Design review of the part built by this model. Coordinates are the model's own, in mm. Face numbers are marked on the shaded views. A direction names the side the tool comes from. Give positions to 0.01 mm unless a question says otherwise; leave off trailing zeros. Write each loop counter-clockwise with the first axis right and the second up, starting at its lowest first coordinate (ties: lowest second). Pieces come first, ordered by that corner, then holes. Notation, with made-up numbers: (-13, 8) - (41, 8) arc R14 ccw to (41, 29) - close; hole circle Ø2 at (84, 80.5). An arc over 180 degrees is marked (long way). Use a Markdown table: item, result. Add a question column.
```python
from build123d import *

# Parameters (mm, degrees)
SKETCH1_R                                           = 35
BOSS_EXTRUDE1_DEPTH                                 = 12
BOSS_EXTRUDE2_START                                 = -4
SKETCH2_R                                           = 35
SKETCH2_R_2                                         = 17.5
BOSS_EXTRUDE2_DEPTH                                 = 4
SKETCH3_W                                           = 20
SKETCH3_H                                           = 20
BOSS_EXTRUDE3_DEPTH                                 = 5.5
CIRPATTERN1_COUNT                                   = 4
CUT_EXTRUDE1_REACH                                  = 123.475
SKETCH4_R                                           = 2.5
FILLET2_R                                           = 10
SKETCH5_R                                           = 35
SKETCH5_R_2                                         = 17.5
BOSS_EXTRUDE4_DEPTH                                 = 6
CSK_FOR_M3_COUNTERSUNK_FLAT_HEAD_SCREW1_D           = 3.4
CSK_FOR_M3_COUNTERSUNK_FLAT_HEAD_SCREW1_CSINK_D     = 6.3
CSK_FOR_M3_COUNTERSUNK_FLAT_HEAD_SCREW1_CSINK_ANGLE = 90
CHAMFER1_SIZE                                       = 1
CHAMFER2_SIZE                                       = 1


with BuildPart() as part:
    # Sketch1 → Boss-Extrude1 (new body)
    with BuildSketch(Plane.XY):
        with BuildLine():
            Line((43.874821937, -10), (85, -10))
            Line((85, -10), (85, 10))
            Line((85, 10), (43.874821937, 10))
            ThreePointArc((43.874821937, 10), (31.819805153, 31.819805153), (10, 43.874821937))
            Line((10, 43.874821937), (10, 85))
            Line((10, 85), (-10, 85))
            Line((-10, 85), (-10, 43.874821937))
            ThreePointArc((-10, 43.874821937), (-31.819805153, 31.819805153), (-43.874821937, 10))
            Line((-43.874821937, 10), (-85, 10))
            Line((-85, 10), (-85, -10))
            Line((-85, -10), (-43.874821937, -10))
            ThreePointArc((-43.874821937, -10), (-31.819805153, -31.819805153), (-10, -43.874821937))
            Line((-10, -43.874821937), (-10, -85))
            Line((-10, -85), (10, -85))
            Line((10, -85), (10, -43.874821937))
            ThreePointArc((10, -43.874821937), (31.819805153, -31.819805153), (43.874821937, -10))
        make_face()
        Circle(SKETCH1_R, mode=Mode.SUBTRACT)
    extrude(amount=BOSS_EXTRUDE1_DEPTH)

    # Sketch2 → Boss-Extrude2 (add)
    with BuildSketch(Plane.XY.offset(12).offset(BOSS_EXTRUDE2_START)):
        Circle(SKETCH2_R)
        Circle(SKETCH2_R_2, mode=Mode.SUBTRACT)
    extrude(amount=BOSS_EXTRUDE2_DEPTH)

    # Sketch3 → Boss-Extrude3 (add)
    with BuildSketch(Plane.XY):
        with Locations((0, 75)):
            Rectangle(SKETCH3_W, SKETCH3_H)
    boss_extrude3 = extrude(amount=-BOSS_EXTRUDE3_DEPTH)

    # CirPattern1: Boss-Extrude3 ×4 about axis
    cirpattern1_axis = Axis((0, 0, 0), (0, 0, 1))
    for i in range(1, CIRPATTERN1_COUNT):
        add(boss_extrude3.rotate(cirpattern1_axis, i * 360 / CIRPATTERN1_COUNT))

    # Sketch4 → Cut-Extrude1 (cut, up to next)
    with BuildSketch(Plane(origin=(0, 0, -5.5), x_dir=(-1, 0, 0), z_dir=(0, 0, -1)), mode=Mode.PRIVATE) as cut_extrude1_sk1:
        with Locations((0, 75)):
            Circle(SKETCH4_R)
    cut_extrude1_tool1 = extrude(cut_extrude1_sk1.sketch, amount=-CUT_EXTRUDE1_REACH, mode=Mode.PRIVATE) & part.part
    # Sketch4 → Cut-Extrude1 (cut, up to next)
    with BuildSketch(Plane(origin=(0, 0, -5.5), x_dir=(-1, 0, 0), z_dir=(0, 0, -1)), mode=Mode.PRIVATE) as cut_extrude1_sk2:
        with Locations((-75, 0)):
            Circle(SKETCH4_R)
    cut_extrude1_tool2 = extrude(cut_extrude1_sk2.sketch, amount=-CUT_EXTRUDE1_REACH, mode=Mode.PRIVATE) & part.part
    # Sketch4 → Cut-Extrude1 (cut, up to next)
    with BuildSketch(Plane(origin=(0, 0, -5.5), x_dir=(-1, 0, 0), z_dir=(0, 0, -1)), mode=Mode.PRIVATE) as cut_extrude1_sk3:
        with Locations((0, -75)):
            Circle(SKETCH4_R)
    cut_extrude1_tool3 = extrude(cut_extrude1_sk3.sketch, amount=-CUT_EXTRUDE1_REACH, mode=Mode.PRIVATE) & part.part
    # Sketch4 → Cut-Extrude1 (cut, up to next)
    with BuildSketch(Plane(origin=(0, 0, -5.5), x_dir=(-1, 0, 0), z_dir=(0, 0, -1)), mode=Mode.PRIVATE) as cut_extrude1_sk4:
        with Locations((75, 0)):
            Circle(SKETCH4_R)
    cut_extrude1_tool4 = extrude(cut_extrude1_sk4.sketch, amount=-CUT_EXTRUDE1_REACH, mode=Mode.PRIVATE) & part.part
    add(cut_extrude1_tool1.solids().sort_by_distance((0, 75, -5.5))[0], mode=Mode.SUBTRACT)
    add(cut_extrude1_tool2.solids().sort_by_distance((75, 0, -5.5))[0], mode=Mode.SUBTRACT)
    add(cut_extrude1_tool3.solids().sort_by_distance((0, -75, -5.5))[0], mode=Mode.SUBTRACT)
    add(cut_extrude1_tool4.solids().sort_by_distance((-75, 0, -5.5))[0], mode=Mode.SUBTRACT)

    # Fillet2
    fillet2_edges = [part.edges().sort_by_distance(p)[0] for p in [
        (10, -43.874821937, 6),
        (-10, -43.874821937, 6),
        (-43.874821937, -10, 6),
        (-43.874821937, 10, 6),
        (-10, 43.874821937, 6),
        (10, 43.874821937, 6),
        (43.874821937, 10, 6),
        (43.874821937, -10, 6),
    ]]
    fillet(fillet2_edges, radius=FILLET2_R)

    # Sketch5 → Boss-Extrude4 (add)
    with BuildSketch(Plane.XY.offset(12)):
        Circle(SKETCH5_R)
        Circle(SKETCH5_R_2, mode=Mode.SUBTRACT)
    extrude(amount=BOSS_EXTRUDE4_DEPTH)

    # CSK for M3 Countersunk Flat Head Screw1 (through all)
    with Locations(Plane(origin=(-15.5, 15.5, 8), x_dir=(-1, 0, 0), z_dir=(0, 0, -1))):
        with Locations((0, 0), (-31, 0), (-31, -31), (0, -31)):
            CounterSinkHole(CSK_FOR_M3_COUNTERSUNK_FLAT_HEAD_SCREW1_D / 2, CSK_FOR_M3_COUNTERSUNK_FLAT_HEAD_SCREW1_CSINK_D / 2, counter_sink_angle=CSK_FOR_M3_COUNTERSUNK_FLAT_HEAD_SCREW1_CSINK_ANGLE)

    # Chamfer1
    chamfer1_edges = [part.edges().sort_by_distance(p)[0] for p in [
        (85, 0, 12),
        (-58.117376915, 10, 0),
        (-68.117376915, 10, 12),
        (-31.819805153, 31.819805153, 0),
        (-31.819805153, 31.819805153, 12),
        (-31.819805153, -31.819805153, 0),
        (-31.819805153, -31.819805153, 12),
        (68.117376915, 10, 12),
        (-10, -58.117376915, 0),
        (-10, -68.117376915, 12),
        (31.819805153, -31.819805153, 0),
        (31.819805153, -31.819805153, 12),
        (58.117376915, -10, 0),
        (68.117376915, -10, 12),
        (31.819805153, 31.819805153, 0),
        (31.819805153, 31.819805153, 12),
        (10, 58.117376915, 0),
        (10, 68.117376915, 12),
        (-45.593993082, 11.742771762, 0),
        (-45.593993082, 11.742771762, 12),
        (-11.742771762, 45.593993082, 0),
        (-11.742771762, 45.593993082, 12),
        (-45.593993082, -11.742771762, 0),
        (-45.593993082, -11.742771762, 12),
        (-11.742771762, -45.593993082, 0),
        (-11.742771762, -45.593993082, 12),
        (11.742771762, -45.593993082, 0),
        (11.742771762, -45.593993082, 12),
        (45.593993082, -11.742771762, 0),
        (45.593993082, -11.742771762, 12),
        (45.593993082, 11.742771762, 0),
        (45.593993082, 11.742771762, 12),
        (11.742771762, 45.593993082, 0),
        (11.742771762, 45.593993082, 12),
        (0, 85, 12),
        (-10, 68.117376915, 12),
        (10, -85, 3.25),
        (-10, -85, 3.25),
        (-85, -10, 3.25),
        (-85, 10, 3.25),
        (-10, 85, 3.25),
        (10, 85, 3.25),
        (85, 10, 3.25),
        (85, -10, 3.25),
        (-85, 0, 12),
        (-68.117376915, -10, 12),
        (0, -85, 12),
        (10, -68.117376915, 12),
        (-10, 58.117376915, 0),
        (10, 75, -5.5),
        (0, 65, -5.5),
        (10, 65, -2.75),
        (-10, 75, -5.5),
        (-10, 65, -2.75),
        (0, 85, -5.5),
        (58.117376915, 10, 0),
        (75, -10, -5.5),
        (65, 0, -5.5),
        (65, -10, -2.75),
        (75, 10, -5.5),
        (65, 10, -2.75),
        (85, 0, -5.5),
        (10, -58.117376915, 0),
        (-10, -75, -5.5),
        (0, -65, -5.5),
        (-10, -65, -2.75),
        (10, -75, -5.5),
        (10, -65, -2.75),
        (0, -85, -5.5),
        (-58.117376915, -10, 0),
        (-75, 10, -5.5),
        (-65, 0, -5.5),
        (-65, 10, -2.75),
        (-75, -10, -5.5),
        (-65, -10, -2.75),
        (-85, 0, -5.5),
    ]]
    chamfer(chamfer1_edges, length=CHAMFER1_SIZE)

    # Chamfer2
    chamfer2_edges = [part.edges().sort_by_distance(p)[0] for p in [
        (-35, 0, 18),
        (-17.5, 0, 18),
        (-35, 0, 0),
        (-17.5, 0, 8),
    ]]
    chamfer(chamfer2_edges, length=CHAMFER2_SIZE)


solid = part.part
```
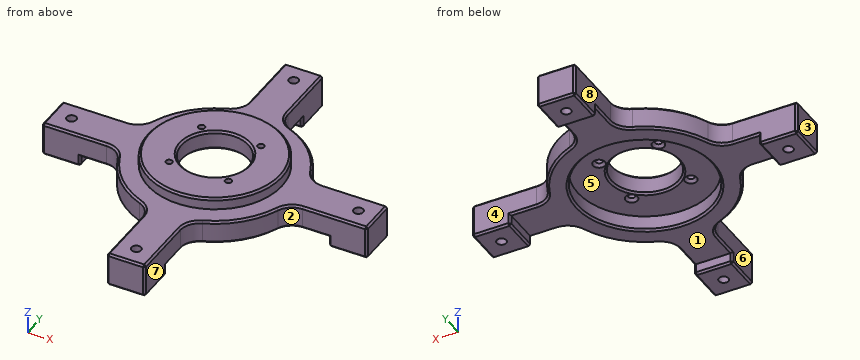
(1) Add section D-D (y = -56.5). State the section outline as (x, z) points, and give its area (3 significant figures).
(2) Tool access review of the marked faces 4, 5, 6, 7 and 8: name each direction out of +Z, -Z, +X, -X, +Y, -Y from which nothing blocks a thin tool from reaching the whole face with its end or side.
(3) Add section A-A (x = -75). State the section outline as (y, z) points, and give its area (4 significant figures).
(4) Mouldability with a two-part tool opening along X and no side actions: class the marked faces 1, 2 and 3 as +X half, -X half, draft (parallel to the pull), parting line (faces both ways), or undercut.
(5) For line 1 along Y through (x, z) = (0, 5.5); line 2 along Y through (x, z) = (-75, 3.5); line 3 along Y through (x, z) = (15.5, 13), list the stretches that pass through material, from the lowest coordinate up.
(6) Insertion check: pin 1 (6.5 mm diameter, centred on x = 75, y = 0, fed in from +Z); pin 2 (10 mm diameter, centred on x = -9, y = -44.5, fed in from -Z); pin 3 (1 mm diameter, centred on y = 36, z = 9, fed in from -X); pin 4 (2 mm diameter, centred on x = 15.5, y = 15.5, fed in from -Z). Each pin has a flat end and moves straight along its axis. Give the tip position at first contact, or say it passes through.
(7) Add section B-B (z = 14). State the section outline as (x, y) points, and give its area (3 significant figures).
Answers follow:
| question | item | result |
|---|---|---|
| 1 | outline | (-10, 1) - (-9, 0) - (9, 0) - (10, 1) - (10, 11) - (9, 12) - (-9, 12) - (-10, 11) - close |
| 1 | area | 238 mm^2 |
| 2 | face 4 | +Z, -Z, +X, +Y |
| 2 | face 5 | -Z |
| 2 | face 6 | +Z, -Z, -X, -Y |
| 2 | face 7 | +Z, -Z, +X, -Y |
| 2 | face 8 | +Z, -Z, -X, +Y |
| 3 | outline | (-10, -4.5) - (-9, -5.5) - (-2.5, -5.5) - (-2.5, 12) - (-9, 12) - (-10, 11) - close; (2.5, -5.5) - (9, -5.5) - (10, -4.5) - (10, 11) - (9, 12) - (2.5, 12) - close |
| 3 | area | 260.5 mm^2 |
| 4 | face 1 | undercut |
| 4 | face 2 | +X half |
| 4 | face 3 | -X half |
| 5 | line 1 | -85 to -77.5, -72.5 to -35, 35 to 72.5, 77.5 to 85 |
| 5 | line 2 | -10 to -2.5, 2.5 to 10 |
| 5 | line 3 | -31.38 to -17.2, -13.8 to -8.12, 8.12 to 13.8, 17.2 to 31.38 |
| 6 | pin 1 | z = 12 |
| 6 | pin 2 | z = 0 |
| 6 | pin 3 | x = -27.65 |
| 6 | pin 4 | through |
| 7 | outline | circle Ø70 at (0, 0); hole circle Ø35 at (0, 0); hole circle Ø3.4 at (-15.5, -15.5); hole circle Ø3.4 at (-15.5, 15.5); hole circle Ø3.4 at (15.5, -15.5); hole circle Ø3.4 at (15.5, 15.5) |
| 7 | area | 2,850 mm^2 |
